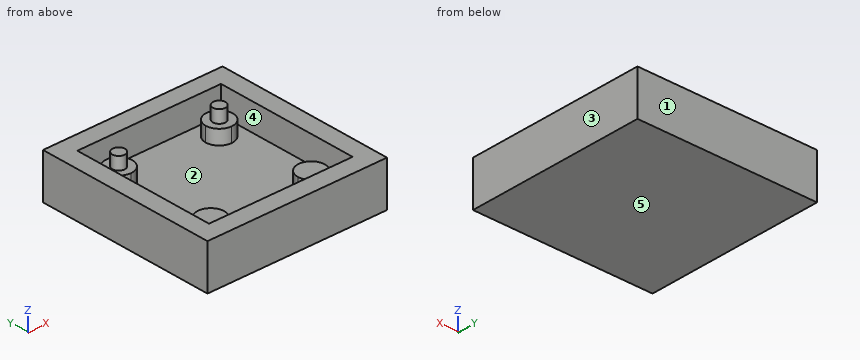
```python
from build123d import *

# Parameters (mm, degrees)
F0_W     = 25.4
F0_H     = 25.4
F1_DEPTH = 6.35
F2_T     = -2.54
F4_DEPTH = 2.032
F5_R     = 0.889
F6_DEPTH = 1.778


with BuildPart() as f1:
    # F0 (on Top) → F1 (new body)
    with BuildSketch(Plane.XY):
        with Locations((-104.38567, -20.633587)):
            Rectangle(F0_W, F0_H)
    extrude(amount=F1_DEPTH)

    # F2
    f2_openings = [f1.faces().sort_by_distance(p)[0] for p in [
        (-104.38567, -20.633587, 6.35),
    ]]
    offset(amount=F2_T, openings=f2_openings)

    # F3 (on face) → F4 (join)
    with BuildSketch(Plane.XY.offset(2.54)):
        with BuildLine():
            ThreePointArc((-111.49767, -15.426587), (-110.150632, -14.868626), (-109.59267, -13.521587))
            Line((-109.59267, -13.521587), (-111.49767, -13.521587))
            Line((-111.49767, -13.521587), (-111.49767, -15.426587))
        make_face()
        with BuildLine():
            Line((-111.49767, -13.521587), (-109.59267, -13.521587))
            ThreePointArc((-109.59267, -13.521587), (-112.844708, -12.174549), (-111.49767, -15.426587))
            Line((-111.49767, -15.426587), (-111.49767, -13.521587))
        make_face()
        with BuildLine():
            ThreePointArc((-95.36867, -13.521587), (-97.27367, -11.616587), (-99.17867, -13.521587))
            Line((-99.17867, -13.521587), (-97.27367, -13.521587))
            Line((-97.27367, -13.521587), (-97.27367, -15.426587))
            ThreePointArc((-97.27367, -15.426587), (-95.926632, -14.868626), (-95.36867, -13.521587))
        make_face()
        with BuildLine():
            Line((-97.27367, -13.521587), (-99.17867, -13.521587))
            ThreePointArc((-99.17867, -13.521587), (-98.620708, -14.868626), (-97.27367, -15.426587))
            Line((-97.27367, -15.426587), (-97.27367, -13.521587))
        make_face()
        with BuildLine():
            Line((-97.27367, -27.745587), (-97.27367, -25.840587))
            ThreePointArc((-97.27367, -25.840587), (-98.620708, -26.398549), (-99.17867, -27.745587))
            Line((-99.17867, -27.745587), (-97.27367, -27.745587))
        make_face()
        with BuildLine():
            ThreePointArc((-95.36867, -27.745587), (-95.926632, -26.398549), (-97.27367, -25.840587))
            Line((-97.27367, -25.840587), (-97.27367, -27.745587))
            Line((-97.27367, -27.745587), (-99.17867, -27.745587))
            ThreePointArc((-99.17867, -27.745587), (-97.27367, -29.650587), (-95.36867, -27.745587))
        make_face()
        with BuildLine():
            Line((-111.49767, -27.745587), (-111.49767, -25.840587))
            ThreePointArc((-111.49767, -25.840587), (-112.844708, -29.092626), (-109.59267, -27.745587))
            Line((-109.59267, -27.745587), (-111.49767, -27.745587))
        make_face()
        with BuildLine():
            ThreePointArc((-109.59267, -27.745587), (-110.150632, -26.398549), (-111.49767, -25.840587))
            Line((-111.49767, -25.840587), (-111.49767, -27.745587))
            Line((-111.49767, -27.745587), (-109.59267, -27.745587))
        make_face()
    extrude(amount=F4_DEPTH)

    # F5 (on face) → F6 (join)
    with BuildSketch(Plane.XY.offset(4.572)):
        with Locations((-111.49767, -13.521587)):
            Circle(F5_R)
        with BuildLine():
            ThreePointArc((-96.38467, -13.521587), (-97.27367, -12.632587), (-98.16267, -13.521587))
            ThreePointArc((-98.16267, -13.521587), (-97.27367, -14.410587), (-96.38467, -13.521587))
        make_face()
    extrude(amount=F6_DEPTH)


solid = f1.part
```
Verification items for the finished model (mm, model axes). Face numbers are marked on the shaded views. A direction names the side the tool comes from. Give positions to 0.01 mm unless a question says otherwise; leave off trailing zeros. Order: outer loops, then holes, each group sorted by start corner. A loop starts at its lowest first (then second) coordinate and runs counter-clockwise, first axis right, second up. Notation, with made-up numbers: M -28,45 L 14,45 A11 cw 14,51 Z; hole C 14,33 d4. An arc over 180 degrees is marked long. Return JSON: item names as keys, results as strings. Group by question number.
1) Section check A-A on z = 3. Record the cut outline in (x, y) (3 decimals).
2) Section check D-D on x = -108.75. Record the cut outline in (y, z), and give its area (3 significant figures).
3) Mould release check, pull along Y, two halves, no side actions. Record for the marked faces 1, 2 and 3: pulls with the +Y half, pulls with the -Y half, needs draft (parallel to the pull), parting line crosses it, or undercut.
4) Section check B-B on z = 5.25. Record the cut outline in (x, y).
5) Scan lines: line 1 (X direction, y = -24.75, z = 3.5); line 2 (Y direction, x = -113, z = 4); line 3 (Y direction, x = -114, z = 5.25). Record each from-to range of solid material in increasing order.
6) Section check C-C on y = -22.75. Record the cut outline in (x, z), and give its area (3 significant figures).
7) Go/stop test with flat-tipped pins: pin 1 Ø1.9 at (x, y) = (-97.5, -27) entering from +Z; pin 2 Ø10 at (x, y) = (-107.5, -21.5) entering from +Z. Record where each tip stops, or that it passes through.
8) Access from +Z, -Z, +X, -X, +Y, -Y to the whole of each face (thin tool, end or side, straight path). Record for the marked faces 4 and 5.
Answer block:
{
 "1": {"outline": "M -117.086,-33.334 L -91.686,-33.334 L -91.686,-7.934 L -117.086,-7.934 Z; C -111.498,-13.522 d3.81; M -111.498,-25.841 A1.905 ccw long -109.593,-27.746 A1.905 ccw Z; M -99.179,-27.746 A1.905 ccw -95.369,-27.746 A1.905 ccw -97.274,-25.841 A1.905 ccw Z; C -97.274,-13.522 d3.81; hole M -114.546,-30.794 L -94.226,-30.794 L -94.226,-10.474 L -114.546,-10.474 Z"},
 "2": {"outline": "M -33.33,0 L -7.93,0 L -7.93,6.35 L -10.47,6.35 L -10.47,2.54 L -30.79,2.54 L -30.79,6.35 L -33.33,6.35 Z", "area": "83.9 mm^2"},
 "3": {"face 1": "pulls with the +Y half", "face 2": "undercut", "face 3": "needs draft"},
 "4": {"outline": "M -117.09,-33.33 L -91.69,-33.33 L -91.69,-7.93 L -117.09,-7.93 Z; C -111.5,-13.52 d1.78; C -97.27,-13.52 d1.78; hole M -114.55,-30.79 L -94.23,-30.79 L -94.23,-10.47 L -114.55,-10.47 Z"},
 "5": {"line 1": "x = -117.09 to -114.55, -94.23 to -91.69", "line 2": "y = -33.33 to -30.79, -28.92 to -26.57, -14.69 to -12.35, -10.47 to -7.93", "line 3": "y = -33.33 to -30.79, -10.47 to -7.93"},
 "6": {"outline": "M -117.09,0 L -91.69,0 L -91.69,6.35 L -94.23,6.35 L -94.23,2.54 L -114.55,2.54 L -114.55,6.35 L -117.09,6.35 Z", "area": "83.9 mm^2"},
 "7": {"pin 1": "stops at z = 4.57", "pin 2": "stops at z = 2.54"},
 "8": {"face 4": "+Z", "face 5": "-Z, +X, -X, +Y, -Y"}
}
